Design review of the part built by this model. Coordinates are the model's own, in mm. A direction names the side the tool comes from. Give positions to 0.01 mm unless a question says otherwise; leave off trailing zeros. Order: outer loops, then holes, each group sorted by start corner. A loop starts at its lowest first (then second) coordinate and runs counter-clockwise, first axis right, second up. Notation, with made-up numbers: M 44,46 L 93,46 A25 ccw 93,85 Z; hole C -34.75,56 d6. An arc over 180 degrees is marked long. Answer as a JSON object with one key per item and string values.
from build123d import *

# Parameters (mm, degrees)
ESQUISSE1_R              = 40
ESQUISSE1_R_2            = 25
BOSS_EXTRU_1_DEPTH       = 20
EMPREINTE1_OUTLINE_R     = 25
EMPREINTE1_DEPTH         = 7.5
EMPREINTE1_START         = 12.5
EMPREINTE1_2_OUTLINE_R   = 25
EMPREINTE1_2_DEPTH       = 7.5
EMPREINTE1_START_2       = 7.5
EMPREINTE1_3_OUTLINE_R   = 27
EMPREINTE1_3_OUTLINE_R_2 = 25
EMPREINTE1_3_DEPTH       = 5


# Read off the part's stored shape, not the designer's step: Empreinte1
with BuildPart() as part:
    # Esquisse1 → Boss.-Extru.1 (new body)
    with BuildSketch(Plane(origin=(0, 0, 0), x_dir=(1, 0, 0), z_dir=(0, 1, 0))):
        with Locations(Location((0, 0, 0), (0, 0, 270))):
            Circle(ESQUISSE1_R)
        with Locations(Location((0, 0, 0), (0, 0, 270))):
            Circle(ESQUISSE1_R_2, mode=Mode.SUBTRACT)
    extrude(amount=BOSS_EXTRU_1_DEPTH)

    # Empreinte1 outline → Empreinte1 (cut)
    with BuildSketch(Plane(origin=(0, 0, 0), x_dir=(1, 0, 0), z_dir=(0, 1, 0))):
        with BuildLine():
            ThreePointArc((-15.75, 27.279800219), (-12.676442841, 26.456243061), (-13.5, 23.382685902))
            ThreePointArc((-13.5, 23.382685902), (-23.382685902, 13.5), (-27, 0))
            ThreePointArc((-27, 0), (-29.25, -2.25), (-31.5, 0))
            ThreePointArc((-31.5, 0), (-31.230513133, 4.111575055), (-30.426663528, 8.152799921))
            ThreePointArc((-30.426663528, 8.152799921), (-32.017653786, 10.908475881), (-34.773329746, 9.317485624))
            ThreePointArc((-34.773329746, 9.317485624), (-31.176914536, -18), (-9.317485624, -34.773329746))
            ThreePointArc((-9.317485624, -34.773329746), (-6.561809663, -33.182339489), (-8.152799921, -30.426663528))
            ThreePointArc((-8.152799921, -30.426663528), (-12.05452812, -29.102205274), (-15.75, -27.279800219))
            ThreePointArc((-15.75, -27.279800219), (-16.573557159, -24.20624306), (-13.5, -23.382685902))
            ThreePointArc((-13.5, -23.382685902), (0, -27), (13.5, -23.382685902))
            ThreePointArc((13.5, -23.382685902), (16.573557159, -24.20624306), (15.75, -27.279800219))
            ThreePointArc((15.75, -27.279800219), (12.05452812, -29.102205274), (8.152799921, -30.426663528))
            ThreePointArc((8.152799921, -30.426663528), (6.561809663, -33.182339489), (9.317485624, -34.773329746))
            ThreePointArc((9.317485624, -34.773329746), (31.176914536, -18), (34.773329746, 9.317485624))
            ThreePointArc((34.773329746, 9.317485624), (32.017653786, 10.908475881), (30.426663528, 8.152799921))
            ThreePointArc((30.426663528, 8.152799921), (31.230513133, 4.111575055), (31.5, 0))
            ThreePointArc((31.5, 0), (29.25, -2.25), (27, 0))
            ThreePointArc((27, 0), (23.382685902, 13.5), (13.5, 23.382685902))
            ThreePointArc((13.5, 23.382685902), (12.676442841, 26.456243061), (15.75, 27.279800219))
            ThreePointArc((15.75, 27.279800219), (19.175985014, 24.990630219), (22.273863607, 22.273863607))
            ThreePointArc((22.273863607, 22.273863607), (25.455844123, 22.273863607), (25.455844123, 25.455844123))
            ThreePointArc((25.455844123, 25.455844123), (0, 36), (-25.455844123, 25.455844123))
            ThreePointArc((-25.455844123, 25.455844123), (-25.455844123, 22.273863607), (-22.273863607, 22.273863607))
            ThreePointArc((-22.273863607, 22.273863607), (-19.175985014, 24.990630219), (-15.75, 27.279800219))
        make_face()
        Circle(EMPREINTE1_OUTLINE_R, mode=Mode.SUBTRACT)
    extrude(amount=EMPREINTE1_DEPTH, mode=Mode.SUBTRACT)

    # Empreinte1 2 outline → Empreinte1 2 (cut)
    with BuildSketch(Plane(origin=(0, 0, 0), x_dir=(1, 0, 0), z_dir=(0, 1, 0)).offset(EMPREINTE1_START)):
        with BuildLine():
            ThreePointArc((-15.75, 27.279800219), (-12.676442841, 26.456243061), (-13.5, 23.382685902))
            ThreePointArc((-13.5, 23.382685902), (-23.382685902, 13.5), (-27, 0))
            ThreePointArc((-27, 0), (-29.25, -2.25), (-31.5, 0))
            ThreePointArc((-31.5, 0), (-31.230513133, 4.111575055), (-30.426663528, 8.152799921))
            ThreePointArc((-30.426663528, 8.152799921), (-32.017653786, 10.908475881), (-34.773329746, 9.317485624))
            ThreePointArc((-34.773329746, 9.317485624), (-31.176914536, -18), (-9.317485624, -34.773329746))
            ThreePointArc((-9.317485624, -34.773329746), (-6.561809663, -33.182339489), (-8.152799921, -30.426663528))
            ThreePointArc((-8.152799921, -30.426663528), (-12.05452812, -29.102205274), (-15.75, -27.279800219))
            ThreePointArc((-15.75, -27.279800219), (-16.573557159, -24.20624306), (-13.5, -23.382685902))
            ThreePointArc((-13.5, -23.382685902), (0, -27), (13.5, -23.382685902))
            ThreePointArc((13.5, -23.382685902), (16.573557159, -24.20624306), (15.75, -27.279800219))
            ThreePointArc((15.75, -27.279800219), (12.05452812, -29.102205274), (8.152799921, -30.426663528))
            ThreePointArc((8.152799921, -30.426663528), (6.561809663, -33.182339489), (9.317485624, -34.773329746))
            ThreePointArc((9.317485624, -34.773329746), (31.176914536, -18), (34.773329746, 9.317485624))
            ThreePointArc((34.773329746, 9.317485624), (32.017653786, 10.908475881), (30.426663528, 8.152799921))
            ThreePointArc((30.426663528, 8.152799921), (31.230513133, 4.111575055), (31.5, 0))
            ThreePointArc((31.5, 0), (29.25, -2.25), (27, 0))
            ThreePointArc((27, 0), (23.382685902, 13.5), (13.5, 23.382685902))
            ThreePointArc((13.5, 23.382685902), (12.676442841, 26.456243061), (15.75, 27.279800219))
            ThreePointArc((15.75, 27.279800219), (19.175985014, 24.990630219), (22.273863607, 22.273863607))
            ThreePointArc((22.273863607, 22.273863607), (25.455844123, 22.273863607), (25.455844123, 25.455844123))
            ThreePointArc((25.455844123, 25.455844123), (0, 36), (-25.455844123, 25.455844123))
            ThreePointArc((-25.455844123, 25.455844123), (-25.455844123, 22.273863607), (-22.273863607, 22.273863607))
            ThreePointArc((-22.273863607, 22.273863607), (-19.175985014, 24.990630219), (-15.75, 27.279800219))
        make_face()
        Circle(EMPREINTE1_2_OUTLINE_R, mode=Mode.SUBTRACT)
    extrude(amount=EMPREINTE1_2_DEPTH, mode=Mode.SUBTRACT)

    # Empreinte1 3 outline → Empreinte1 3 (cut)
    with BuildSketch(Plane(origin=(0, 0, 0), x_dir=(1, 0, 0), z_dir=(0, 1, 0)).offset(EMPREINTE1_START_2)):
        Circle(EMPREINTE1_3_OUTLINE_R)
        Circle(EMPREINTE1_3_OUTLINE_R_2, mode=Mode.SUBTRACT)
    extrude(amount=EMPREINTE1_3_DEPTH, mode=Mode.SUBTRACT)


solid = part.part
(1) To check wall thickness, follow L1, parallel to X at y = 17.5, z = 1; L2, parallel to X at y = 8.8, z = 0; L3, parallel to Y at x = 18, z = 23. State the ranges of each line that lie inside material, in increasing order. Write a range as from..to.
Checked values:
{"L1": "x = -39.99..-35.99, -31.27..-27.23, 27.23..31.27, 35.99..39.99", "L2": "x = -40..-27, 27..40", "L3": "y = 7.5..12.5"}
(2) Insertion check: pin 1 (15 mm diameter, centred on x = -25.5, z = 20, fed in from +Y); pin 2 (6 mm diameter, centred on x = 21.5, z = 2, fed in from -Y); pin 3 (10 mm diameter, centred on x = -18, y = 6.5, fed in from +Z); pin 4 (1 mm diameter, centred on x = -5, y = 3, fed in from +Z). Each pin has a flat end and moves straight along its axis. Give the tip position at first contact, or say it passes through.
Checked values:
{"pin 1": "stops at y = 20", "pin 2": "passes through", "pin 3": "stops at z = 37.83", "pin 4": "stops at z = 39.75"}
(3) We need section B-B (z = -4). Write out the cut boundary in (x, y) (1 decimal), plus the area to 3 significant figures.
Checked values:
{"outline": "M -39.8,0 L -35.8,0 L -35.8,7.5 L -31.2,7.5 L -31.2,0 L -26.7,0 L -26.7,20 L -31.2,20 L -31.2,12.5 L -35.8,12.5 L -35.8,20 L -39.8,20 Z; M 26.7,0 L 31.2,0 L 31.2,7.5 L 35.8,7.5 L 35.8,0 L 39.8,0 L 39.8,20 L 35.8,20 L 35.8,12.5 L 31.2,12.5 L 31.2,20 L 26.7,20 Z", "area": "388 mm^2"}
(4) Tool access review of faces 1 (the cylindrical face through (-12.702, 3.698, -26.499)), 2 (the cylindrical face through (19.13, 16.197, -25.026)): name each direction out of +Z, -Z, +X, -X, +Y, -Y from which nothing blocks a thin tool from reaching the whole face with its end or side.
Checked values:
{"face 1": "-Y", "face 2": "+Y"}
(5) We need section A-A (x = 0). Write out the cut boundary in (y, z).
Checked values:
{"outline": "M 0,-40 L 20,-40 L 20,-36 L 12.5,-36 L 12.5,-27 L 7.5,-27 L 7.5,-36 L 0,-36 Z; M 0,27 L 20,27 L 20,40 L 0,40 Z"}
(6) We need section D-D (x = 29.25). Write out the cut boundary in (y, z), plus the area to 3 significant figures.
Checked values:
{"outline": "M 0,-27.28 L 20,-27.28 L 20,2.25 L 12.5,2.25 L 12.5,20.99 L 20,20.99 L 20,27.28 L 0,27.28 L 0,20.99 L 7.5,20.99 L 7.5,2.25 L 0,2.25 Z", "area": "810 mm^2"}
(7) We need section C-C (y = 10.25). Write out the cut boundary in (x, z).
Checked values:
{"outline": "C 0,0 d80; hole C 0,0 d54"}
